from build123d import *

# Parameters (mm, degrees)
BOSS_EXTRUDE1_DEPTH = 36
CUT_EXTRUDE1_REACH  = 21.399
CUT_EXTRUDE2_REACH  = 21.399
BOSS_EXTRUDE2_DEPTH = 2
CUT_EXTRUDE3_REACH  = 21.399
SKETCH5_R           = 1.5
CUT_EXTRUDE4_REACH  = 11
SKETCH6_W           = 5
SKETCH6_H           = 17


with BuildPart() as part:
    # Sketch1 → Boss-Extrude1 (new body)
    with BuildSketch(Plane(origin=(0, 0, 0), x_dir=(1, 0, 0), z_dir=(0, 1, 0))):
        Polygon((0, 0), (11.909668113, 0), (14.399319728, 2.489651615), (17.399319728, 2.489651615), (17.399319728, 21), (19.399319728, 21), (19.399319728, 1.06122449), (15.799319728, 1.06122449), (12.738095238, -2), (10, -2), (10, -9), (0, -9), align=None)
    extrude(amount=BOSS_EXTRUDE1_DEPTH)

    # Sketch2 → Cut-Extrude1 (cut, up to next)
    with BuildSketch(Plane(origin=(19.399319728, 0, 0), x_dir=(0, 0, -1), z_dir=(1, 0, 0)), mode=Mode.PRIVATE) as cut_extrude1_sk1:
        Polygon((3.06122449, 0), (3.06122449, 3), (21, 28.619226488), (21, 0), align=None)
    cut_extrude1_tool1 = extrude(cut_extrude1_sk1.sketch, amount=-CUT_EXTRUDE1_REACH, mode=Mode.PRIVATE) & part.part
    add(cut_extrude1_tool1.solids().sort_by_distance((19.39932, 9.634621, -14.453071))[0], mode=Mode.SUBTRACT)

    # Sketch3 → Cut-Extrude2 (cut, up to next)
    with BuildSketch(Plane(origin=(19.399319728, 0, 0), x_dir=(0, 0, -1), z_dir=(1, 0, 0)), mode=Mode.PRIVATE) as cut_extrude2_sk1:
        with BuildLine():
            Line((5.06122449, 17.745124794), (5.06122449, 30))
            ThreePointArc((5.06122449, 30), (5.354117709, 30.707106781), (6.06122449, 31))
            Line((6.06122449, 31), (13, 31))
            ThreePointArc((13, 31), (13.707106781, 30.707106781), (14, 30))
            Line((14, 30), (14, 27.654723208))
            ThreePointArc((14, 27.654723208), (13.953716951, 27.354017409), (13.819152044, 27.081146772))
            Line((13.819152044, 27.081146772), (6.880376534, 17.171548358))
            ThreePointArc((6.880376534, 17.171548358), (5.76051869, 16.791407843), (5.06122449, 17.745124794))
        make_face()
    cut_extrude2_tool1 = extrude(cut_extrude2_sk1.sketch, amount=-CUT_EXTRUDE2_REACH, mode=Mode.PRIVATE) & part.part
    add(cut_extrude2_tool1.solids().sort_by_distance((19.39932, 25.474687, -8.644546))[0], mode=Mode.SUBTRACT)

    # Sketch4 → Boss-Extrude2 (add)
    with BuildSketch(Plane(origin=(19.399319728, 0, 0), x_dir=(0, 0, -1), z_dir=(1, 0, 0))):
        with BuildLine():
            Line((21, 36), (21, 39))
            ThreePointArc((21, 39), (17, 43), (13, 39))
            Line((13, 39), (13, 36))
            Line((13, 36), (21, 36))
        make_face()
    extrude(amount=-BOSS_EXTRUDE2_DEPTH)

    # Sketch5 → Cut-Extrude3 (cut, up to next)
    with BuildSketch(Plane(origin=(19.399319728, 0, 0), x_dir=(0, 0, -1), z_dir=(1, 0, 0)), mode=Mode.PRIVATE) as cut_extrude3_sk1:
        with Locations((17, 37)):
            Circle(SKETCH5_R)
    cut_extrude3_tool1 = extrude(cut_extrude3_sk1.sketch, amount=-CUT_EXTRUDE3_REACH, mode=Mode.PRIVATE) & part.part
    add(cut_extrude3_tool1.solids().sort_by_distance((19.39932, 37, -17))[0], mode=Mode.SUBTRACT)

    # Sketch6 → Cut-Extrude4 (cut, up to next)
    with BuildSketch(Plane(origin=(0, 0, 0), x_dir=(-1, 0, 0), z_dir=(0, 0, -1)), mode=Mode.PRIVATE) as cut_extrude4_sk1:
        with Locations((-2.5, 16.5)):
            Rectangle(SKETCH6_W, SKETCH6_H)
    cut_extrude4_tool1 = extrude(cut_extrude4_sk1.sketch, amount=-CUT_EXTRUDE4_REACH, mode=Mode.PRIVATE) & part.part
    add(cut_extrude4_tool1.solids().sort_by_distance((2.5, 16.5, 0))[0], mode=Mode.SUBTRACT)


solid = part.part
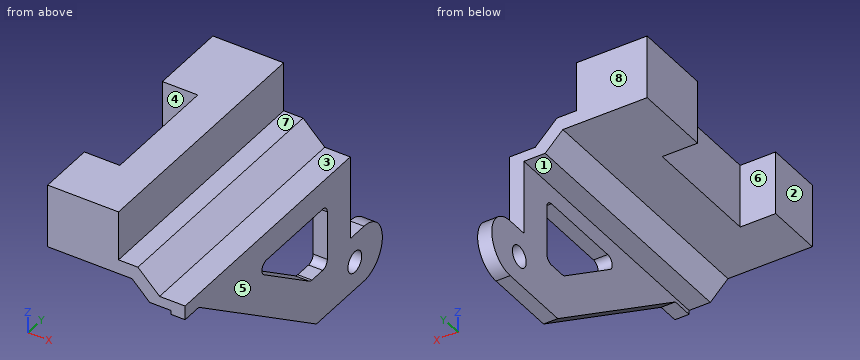
Verification items for the finished model (mm, model axes). Face numbers are marked on the shaded views. A direction names the side the tool comes from. Round coordinates to 2 decimals unless told otherwise and drop trailing zeros. Loops run counter-clockwise (first coordinate to the right, second up) from the corner with the lowest first, then second, coordinate; pieces in that order, holes last. Notation, with made-up numbers: (63.5, 12.5) - (87.5, 12.5) arc R32 cw to (87.5, 39.5) - close; hole circle Ø2 at (-12.75, -16). An arc over 180 degrees is marked (long way). Use a Markdown table: item, result. Add a question column.
1. Section check A-A, the plane x = 2.5. Record the boundary of the cut face in (y, z).
2. Section check C-C, the plane z = 1.25. Record the boundary of the cut face in (x, y).
3. Section check D-D, the plane y = 12. Record the boundary of the cut face in (x, z).
4. Section check B-B, the plane y = 37. Record the boundary of the cut face in (x, z), plus the area to 3 significant figures.
5. Access from +Z, -Z, +X, -X, +Y, -Y to the whole of each face (thin tool, end or side, straight path). Record for the marked faces 1, 2, 3, 4 and 5.
6. Release check for a two-part mould opening along Y. For the marked faces 6, 7 and 8 record: released by +Y, released by -Y, zero draft, split by the parting line, or undercut.
7. Gauge pin test, flat ends, axial feed: pin 1 (1.6 mm diameter, centred on x = 18, z = -9.5, fed in from -Y); pin 2 (4.5 mm diameter, centred on y = 16.5, z = 5, fed in from -X); pin 3 (1 mm diameter, centred on x = 18, y = 28.5, fed in from +Z); pin 4 (1.5 mm diameter, centred on x = 1.5, z = 2.5, fed in from -Y). Record the tip position at first contact, or that the pin passes through.
8. Thickness scan on probe 1 along Z at (x, y) = (8.5, 10); probe 2 along X at (y, z) = (9.5, -4.25); probe 3 along Y at (x, z) = (5.75, 5.75). Record the ranges inside material, lowest first. Write a range as [from, to].
Checks:
| question | item | result |
|---|---|---|
| 1 | outline | (0, 0) - (8, 0) - (8, 9) - (0, 9) - close; (25, 0) - (36, 0) - (36, 9) - (25, 9) - close |
| 2 | outline | (0, 0) - (13.49, 0) - (13.49, 36) - (0, 36) - (0, 25) - (5, 25) - (5, 8) - (0, 8) - close |
| 3 | outline | (5, 0) - (11.91, 0) - (14.4, -2.49) - (17.4, -2.49) - (17.4, -9.36) - (19.4, -9.36) - (19.4, -1.06) - (15.8, -1.06) - (12.74, 2) - (10, 2) - (10, 9) - (5, 9) - close |
| 4 | outline | (17.4, -21) - (19.4, -21) - (19.4, -18.5) - (17.4, -18.5) - close; (17.4, -15.5) - (19.4, -15.5) - (19.4, -13) - (17.4, -13) - close |
| 4 | area | 10.0 mm^2 |
| 5 | face 1 | -Z, -X, +Y, -Y |
| 5 | face 2 | +Z, -Z, -X, +Y, -Y |
| 5 | face 3 | +Z, +X, +Y, -Y |
| 5 | face 4 | +Z, -Z, -X |
| 5 | face 5 | +Z, -Z, +X, +Y, -Y |
| 6 | face 6 | undercut |
| 6 | face 7 | zero draft |
| 6 | face 8 | released by +Y |
| 7 | pin 1 | stops at y = 11.05 |
| 7 | pin 2 | stops at x = 5 |
| 7 | pin 3 | stops at z = -1.06 |
| 7 | pin 4 | stops at y = 0 |
| 8 | probe 1 | z = [0, 9] |
| 8 | probe 2 | x = [17.4, 19.4] |
| 8 | probe 3 | y = [0, 36] |
